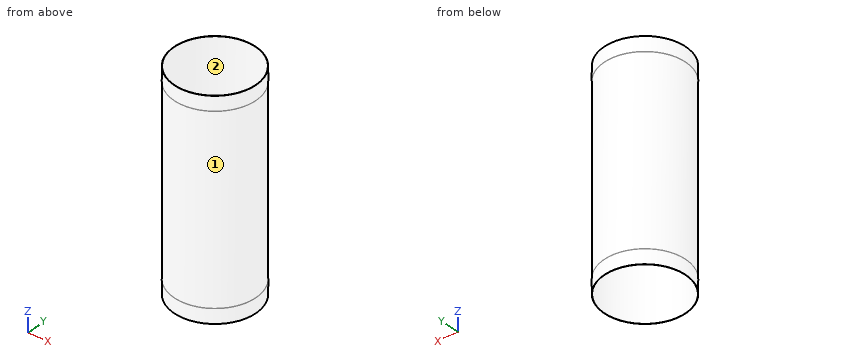
```python
from build123d import *

# Parameters (mm, degrees)
SKETCH1_R      = 216.126
SKETCH1_R_2    = 214.95
EXTRUDE1_DEPTH = 559.8


with BuildPart() as part:
    # Sketch1 → Extrude1 (new body, symmetric)
    with BuildSketch(Plane.XY):
        Circle(SKETCH1_R)
        Circle(SKETCH1_R_2, mode=Mode.SUBTRACT)
    extrude(amount=EXTRUDE1_DEPTH, both=True)

    # Sketch2 → Cut-Revolve1 (revolve, cut)
    with BuildSketch(Plane(origin=(0, 0, 0), x_dir=(1, 0, 0), z_dir=(0, 1, 0)), mode=Mode.PRIVATE) as cut_revolve1_sk:
        Polygon((216.126, 484.8), (215.905, 482.8), (215.905, -482.8), (216.126, -484.8), align=None)
    revolve(cut_revolve1_sk.sketch.rotate(Axis((0, 0, -624.558028957), (0, 0, 1)), 180), axis=Axis((0, 0, -624.558028957), (0, 0, 1)), mode=Mode.SUBTRACT)  # turned: the seam where the file's is


solid = part.part
```
Part model, mm, in its own coordinate system. Face numbers are marked on the shaded views. Give positions to 0.01 mm unless a question says otherwise; leave off trailing zeros. Order: outer loops, then holes, each group sorted by start corner. A loop starts at its lowest first (then second) coordinate and runs counter-clockwise, first axis right, second up. Notation, with made-up numbers: M 75.5,43 L 114.5,43 A12 cw 114.5,60 Z; hole C 3,8 d10. An arc over 180 degrees is marked long. Use a Markdown table: item, result. Add a question column.
(1) Saw through at A-A, the plane y = 0. Give the cut face in (x, z) (3 decimals), and give its area (3 significant figures).
(2) Saw through at C-C, the plane z = 164. Give the cut face in (x, y) (3 decimals), and give its area (3 significant figures).
(3) Drop flat-ended pins along their axis: P1, Ø12, axis at x = -168.5, z = 391.5, coming from the +Y side; P2, Ø1, axis at y = -129, z = 170, coming from the -X side; P3, Ø1.5, axis at x = -81.5, z = 329.5, coming from the +Y side. Give the stop position or say it passes through.
(4) Probe line 1 along Y through (x, z) = (0, 89) (3 decimals); line 2 along X through (y, z) = (-51, -109.5); line 3 along X through (y, z) = (41.5, 61.5). List the from-to ranges inside material, lowest first. Write a range as [from, to].
(5) Mould opens along X. For the marked faces 1 and 2 say: +X half, -X half, draft (parallel to the pull), parting line (faces both ways), or undercut.
Answer key:
| question | item | result |
|---|---|---|
| 1 | outline | M -216.126,-559.8 L -214.95,-559.8 L -214.95,559.8 L -216.126,559.8 L -216.126,484.8 L -215.905,482.8 L -215.905,-482.8 L -216.126,-484.8 Z; M 214.95,-559.8 L 216.126,-559.8 L 216.126,-484.8 L 215.905,-482.8 L 215.905,482.8 L 216.126,484.8 L 216.126,559.8 L 214.95,559.8 Z |
| 1 | area | 2,210 mm^2 |
| 2 | outline | C 0,0 d431.81; hole C 0,0 d429.9 |
| 2 | area | 1,290 mm^2 |
| 3 | P1 | y = 142.16 |
| 3 | P2 | x = -173.5 |
| 3 | P3 | y = 200.24 |
| 4 | line 1 | [-215.905, -214.95], [214.95, 215.905] |
| 4 | line 2 | [-209.8, -208.81], [208.81, 209.8] |
| 4 | line 3 | [-211.88, -210.91], [210.91, 211.88] |
| 5 | face 1 | parting line |
| 5 | face 2 | undercut |
